Geometry: final body of the model. Coordinates: model frame, mm. Give positions to 0.01 mm unless a question says otherwise; leave off trailing zeros. Write each loop counter-clockwise with the first axis right and the second up, starting at its lowest first coordinate (ties: lowest second). Pieces come first, ordered by that corner, then holes. Notation, with made-up numbers: (7, -13) -> (19, -13) arc R22 ccw to (19, -6) -> close; hole circle Ø6 at (59, -38). An arc over 180 degrees is marked (long way). Answer as a JSON object with one key per item and string values.
from build123d import *

# Parameters (mm, degrees)
BOSS_EXTRUDE1_DEPTH = 0.762
FILLET1_R           = 0.762


with BuildPart() as part:
    # Sketch1 → Boss-Extrude1 (new body)
    with BuildSketch(Plane.XY):
        with BuildLine():
            Line((-27.305, 9.525), (27.305, 9.525))
            ThreePointArc((27.305, 9.525), (32.693153673, 7.293153673), (34.925, 1.905))
            Line((34.925, 1.905), (34.925, -2.636770687))
            ThreePointArc((34.925, -2.636770687), (32.855798288, -6.728407727), (28.333860759, -7.486807614))
            ThreePointArc((28.333860759, -7.486807614), (28.089406783, -7.411002579), (27.84475, -7.335854667))
            Line((27.84475, -7.335854667), (27.84475, 0))
            ThreePointArc((27.84475, 0), (23.8125, 4.03225), (19.78025, 0))
            Line((19.78025, 0), (19.78025, -5.251483323))
            ThreePointArc((19.78025, -5.251483323), (0, -3.175), (-19.78025, -5.251483323))
            Line((-19.78025, -5.251483323), (-19.78025, 0))
            ThreePointArc((-19.78025, 0), (-23.8125, 4.03225), (-27.84475, 0))
            Line((-27.84475, 0), (-27.84475, -7.335854667))
            ThreePointArc((-27.84475, -7.335854667), (-28.089406783, -7.411002579), (-28.333860759, -7.486807614))
            ThreePointArc((-28.333860759, -7.486807614), (-32.855798288, -6.728407727), (-34.925, -2.636770687))
            Line((-34.925, -2.636770687), (-34.925, 1.905))
            ThreePointArc((-34.925, 1.905), (-32.693153673, 7.293153673), (-27.305, 9.525))
        make_face()
    extrude(amount=BOSS_EXTRUDE1_DEPTH)

    # Fillet1
    fillet1_edges = [part.edges().sort_by_distance(p)[0] for p in [
        (27.84475, -7.335854667, 0.381),
        (19.78025, -5.251483323, 0.381),
        (-19.78025, -5.251483323, 0.381),
        (-27.84475, -7.335854667, 0.381),
    ]]
    fillet(fillet1_edges, radius=FILLET1_R)


solid = part.part
Q1. Cut plane B-B (x = -15). Return the cut outline in (y, z) (3 decimals).
Values:
{"outline": "(-4.364, 0) -> (9.525, 0) -> (9.525, 0.762) -> (-4.364, 0.762) -> close"}
Q2. Mould query, pull axis X, two halves, no side actions, for faces 1 (the cylindrical face through (32.634, 7.352, 0.376)), 2 (the flat face through (0, 3, 0.762)), 3 (the cylindrical face through (-23.72, 4.03, 0.38)). Classes: pulls with the +X half, pulls with the -X half, needs draft (parallel to the pull), parting line crosses it, or undercut.
Values:
{"face 1": "pulls with the +X half", "face 2": "needs draft", "face 3": "undercut"}
Q3. Material intervals for L1, parallel to X at y = -0.5, z = 0.5 (3 decimals); L2, parallel to X at y = 3.25, z = 0.3; L3, parallel to X at y = -7, z = 0.15, sorted ascending. Write a range as from..to.
Values:
{"L1": "-34.925..-27.845, -19.78..19.78, 27.845..34.925", "L2": "-34.81..-26.2, -21.43..21.43, 26.2..34.81", "L3": "-32.45..-27.88, 27.88..32.45"}
Q4. Cut plane A-A (x = 13). Return the cut outline in (y, z) (3 decimals), and give its area (3 significant figures).
Values:
{"outline": "(-4.066, 0) -> (9.525, 0) -> (9.525, 0.762) -> (-4.066, 0.762) -> close", "area": "10.4 mm²"}
